Build history of the part. All positions in model axes, mm. Face numbers are marked on the shaded views. A direction names the side the tool comes from. Round coordinates to 2 decimals unless told otherwise and drop trailing zeros. Write each loop counter-clockwise with the first axis right and the second up, starting at its lowest first coordinate (ties: lowest second). Pieces come first, ordered by that corner, then holes. Notation, with made-up numbers: M 78.25,77.5 L 121.25,77.5 A24 cw 121.25,91.5 Z; hole C 60.25,18 d7. An arc over 180 degrees is marked long. One line per item, written item: value. Start each with the question number.
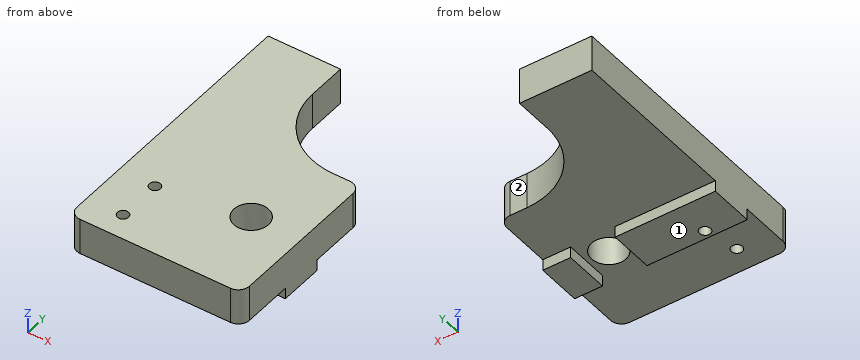
```python
from build123d import *

# Parameters (mm, degrees)
PAD_DEPTH       = 6.5
SKETCH001_W     = 18
SKETCH001_H     = 8
SKETCH001_W_2   = 5
PAD001_DEPTH    = 2
SKETCH002_R     = 3.1
POCKET_DEPTH    = 6.501
SKETCH003_R     = 1
POCKET001_DEPTH = 8.501
FILLET_R        = 13
FILLET001_R     = 2


with BuildPart() as part:
    # Sketch → Pad (new body)
    with BuildSketch(Plane.XY):
        Polygon((0, -15), (31, -15), (31, 15), (13, 15), (13, 35), (0, 35), align=None)
    extrude(amount=PAD_DEPTH)

    # Sketch001 (on Face7 of Pad) → Pad001 (join)
    with BuildSketch(Plane(origin=(0, 0, 0), x_dir=(1, 0, 0), z_dir=(0, 0, -1))):
        with Locations((9, 0)):
            Rectangle(SKETCH001_W, SKETCH001_H)
        with Locations((28.5, 0)):
            Rectangle(SKETCH001_W_2, SKETCH001_H)
    extrude(amount=PAD001_DEPTH)

    # Sketch002 (on Face4 of Pad001) → Pocket (cut, through all)
    with BuildSketch(Plane(origin=(0, 0, 0), x_dir=(1, 0, 0), z_dir=(0, 0, -1))):
        with Locations((22, 0)):
            Circle(SKETCH002_R)
    extrude(amount=-POCKET_DEPTH, mode=Mode.SUBTRACT)

    # Sketch003 (on Face5 of Pocket) → Pocket001 (cut, through all)
    with BuildSketch(Plane.XY.offset(6.5)):
        with Locations((6.5, -10.5)):
            Circle(SKETCH003_R)
        with Locations((6.5, -2.5)):
            Circle(SKETCH003_R)
    extrude(amount=-POCKET001_DEPTH, mode=Mode.SUBTRACT)

    # Fillet
    fillet_edges = [part.edges().sort_by_distance(p)[0] for p in [
        (13, 15, 3.25),
    ]]
    fillet(fillet_edges, radius=FILLET_R)

    # Fillet001
    fillet001_edges = [part.edges().sort_by_distance(p)[0] for p in [
        (31, 15, 3.25),
        (31, -15, 3.25),
        (0, -15, 3.25),
    ]]
    fillet(fillet001_edges, radius=FILLET001_R)


solid = part.part
```
Item 1: Cut at D-D, the plane x = 3. Write the cut outline in (y, z).
Item 2: Drop flat-ended pins along their axis: pin 1 (0.6 mm diameter, centred on x = 29.5, z = -0.5, fed in from -Y); pin 2 (1.6 mm diameter, centred on y = -2, z = -1, fed in from -X); pin 3 (7 mm diameter, centred on x = 22, y = 0, fed in from -Z); pin 4 (1 mm diameter, centred on x = 6, z = -1.5, fed in from +Y). Give the stop position or say it passes through.
Item 3: Which spindle directions (+Z, -Z, +X, -X, +Y, -Y) get a long thin tool onto all of the face, cutting with end or side? Do the marked faces 1 and 2. Say none if no direction does.
Item 4: Cut at A-A, the plane y = -10.5. Write the cut outline in (x, z), plus the area to 4 significant figures.
Item 5: Drill centre lines: line 1 (Y direction, x = 6.5, z = 4.5); line 2 (Z direction, x = 11.5, y = 14); line 3 (Y direction, x = 22, z = 4.5). Where is each one in solid material? Low to high.
Item 6: Cut at B-B, the plane z = 5. Write the cut outline in (x, y), plus the area to 3 significant figures.
Item 7: Cut at C-C, the plane x = 7. Write the cut outline in (y, z).
Computed values:
1. outline: M -15,0 L -4,0 L -4,-2 L 4,-2 L 4,0 L 35,0 L 35,6.5 L -15,6.5 Z
2. pin 1: stops at y = -4
2. pin 2: stops at x = 0
2. pin 3: stops at z = 0
2. pin 4: stops at y = 4
3. face 1: -Z, +X, -X, +Y, -Y
3. face 2: +Z, -Z, +X, +Y
4. outline: M 0,0 L 5.5,0 L 5.5,6.5 L 0,6.5 Z; M 7.5,0 L 31,0 L 31,6.5 L 7.5,6.5 Z
4. area: 188.5 mm2
5. line 1: y = -15 to -11.5, -9.5 to -3.5, -1.5 to 35
5. line 2: z = 0 to 6.5
5. line 3: y = -15 to -3.1, 3.1 to 15.63
6. outline: M 0,-13 A2 ccw 2,-15 L 29,-15 A2 ccw 31,-13 L 31,13 A2 ccw 29,15 L 26,15 A13 cw 13,28 L 13,35 L 0,35 Z; hole C 6.5,-10.5 d2; hole C 6.5,-2.5 d2; hole C 22,0 d6.2
6. area: 1,190 mm2
7. outline: M -15,0 L -11.37,0 L -11.37,6.5 L -15,6.5 Z; M -9.63,0 L -4,0 L -4,-2 L -3.37,-2 L -3.37,6.5 L -9.63,6.5 Z; M -1.63,-2 L 4,-2 L 4,0 L 35,0 L 35,6.5 L -1.63,6.5 Z
